from build123d import *

# Parameters (mm, degrees)
BOSS_EXTRUDE1_DEPTH = 11.5
REVOLVE1_ANGLE      = 180
FILLET1_R           = 2


with BuildPart() as part:
    # Sketch1 → Boss-Extrude1 (new body)
    with BuildSketch(Plane.XY):
        Polygon((-9, 2.8), (0, 2.8), (0, -2.8), (-9, -2.8), (-9, -4.8), (2, -4.8), (2, 4.8), (-9, 4.8), align=None)
    extrude(amount=BOSS_EXTRUDE1_DEPTH)

    # Sketch2 → Revolve1 (revolve)
    with BuildSketch(Plane.XZ.offset(-2.8)):
        with BuildLine():
            Line((-6, 4.25), (-6, 7.25))
            ThreePointArc((-6, 7.25), (-7.5, 5.75), (-6, 4.25))
        make_face()
    revolve1 = revolve(axis=Axis((-6, 2.8, 4.25), (0, 0, 1)), revolution_arc=REVOLVE1_ANGLE)

    # Mirror1: Revolve1 across plane
    add(revolve1.mirror(Plane.ZX))

    # Fillet1
    fillet1_edges = [part.edges().sort_by_distance(p)[0] for p in [
        (2, 4.8, 5.75),
        (2, -4.8, 5.75),
        (0, -2.8, 5.75),
        (0, 2.8, 5.75),
    ]]
    fillet(fillet1_edges, radius=FILLET1_R)


solid = part.part
Design review of the part built by this model. Coordinates are the model's own, in mm. A direction names the side the tool comes from. Coordinates: 2 decimals unless noted, no trailing zeros. Order: outer loops, then holes, each group sorted by start corner. A loop starts at its lowest first (then second) coordinate and runs counter-clockwise, first axis right, second up. Notation, with made-up numbers: M -31.5,64.5 L -7.5,64.5 A18 ccw -7.5,87.5 Z; hole C 36.5,56 d8. An arc over 180 degrees is marked long. Use a Markdown table: item, result.
(1) For P1, Ø5, axis at y = -1, z = 5.5, coming from the -X side; P2, Ø3, axis at x = -8, y = 0.5, coming from the -Z side, all flat-tipped, find the tip position at first contact; note any pin that passes through.
Worked answers:
| item | result |
|---|---|
| P1 | stops at x = -9 |
| P2 | passes through |
(2) Add section D-D (x = -0.5). Give the boundary of the cut face in (y, z).
Worked answers:
| item | result |
|---|---|
| outline | M -4.8,0 L -2.12,0 L -2.12,11.5 L -4.8,11.5 Z; M 2.12,0 L 4.8,0 L 4.8,11.5 L 2.12,11.5 Z |
(3) Add section A-A (x = -7.75). Give the boundary of the cut face in (y, z).
Worked answers:
| item | result |
|---|---|
| outline | M -4.8,0 L -2.8,0 L -2.8,11.5 L -4.8,11.5 Z; M 2.8,0 L 4.8,0 L 4.8,11.5 L 2.8,11.5 Z |
(4) Add section C-C (y = 1.5). Give the boundary of the cut face in (x, z).
Worked answers:
| item | result |
|---|---|
| outline | C -6,5.75 d1.5; M -0.13,0 L 2,0 L 2,11.5 L -0.13,11.5 Z |
(5) Wall thickness on probe 1 along Y at (x, z) = (-8, 5.75); probe 2 along X at (y, z) = (0.25, 4.25); probe 3 along Y at (x, z) = (-0.5, 3): over which ranges is each line inside the solid? List them lowest first.
Worked answers:
| item | result |
|---|---|
| probe 1 | y = -4.8 to -2.8, 2.8 to 4.8 |
| probe 2 | x = 0 to 2 |
| probe 3 | y = -4.8 to -2.12, 2.12 to 4.8 |
(6) Draft analysis for pull direction Y (two halves, no side actions). For faces 5 (the flat face through (-2, -3, 11.5)), 6 (the cylindrical face through (1.4, 4.23, 5.83)), 7 (the cylindrical face through (1.4, -4.23, 5.83)), 8 (the flat face through (-4.8, 2.8, 6.9)), state which applies: released by +Y, released by -Y, zero draft, split by the parting line, or undercut.
Worked answers:
| item | result |
|---|---|
| face 5 | zero draft |
| face 6 | released by +Y |
| face 7 | released by -Y |
| face 8 | undercut |
(7) For faces 1 (the flat face through (0, 0, 6)), 2 (the flat face through (-9, 4, 6)), 3 (the cylindrical face through (-0.6, 2.23, 5.83)), 4 (the flat face through (-5, -2.8, 4)), list the 3-axis set-ups (+Z, -Z, +X, -X, +Y, -Y) from which the entire face can be reached by the end or side of a thin tool; tool diameter is ignored.
Worked answers:
| item | result |
|---|---|
| face 1 | +Z, -Z, -X |
| face 2 | +Z, -Z, -X, +Y, -Y |
| face 3 | +Z, -Z |
| face 4 | none |
(8) Add section B-B (z = 7.75). Give the boundary of the cut face in (x, y).
Worked answers:
| item | result |
|---|---|
| outline | M -9,-4.8 L 0,-4.8 A2 ccw 2,-2.8 L 2,2.8 A2 ccw 0,4.8 L -9,4.8 L -9,2.8 L -2,2.8 A2 cw 0,0.8 L 0,-0.8 A2 cw -2,-2.8 L -9,-2.8 Z |
